The listing builds one solid part. Answer for the finished solid, in the listing's coordinates (mm). A direction names the side the tool comes from. Round coordinates to 2 decimals unless told otherwise and drop trailing zeros. Order: outer loops, then holes, each group sorted by start corner. A loop starts at its lowest first (then second) coordinate and runs counter-clockwise, first axis right, second up. Notation, with made-up numbers: M 36.25,64 L 63.25,64 A22 cw 63.25,100 Z; hole C 24,-9.75 d5. An arc over 180 degrees is marked long. Write item = value, one per line. Start each with the question number.
(1) A cutting plane is placed at C-C, the plane y = 39. Determine the outline of the cut face in (x, z), and give its area (3 significant figures).
(2) A cutting plane is placed at B-B, the plane y = 3. Determine the outline of the cut face in (x, z).
(3) Each of these flat-tipped pins is pushed along its axis until it touches: pin 1 (6 mm diameter, centred on x = 4.5, y = 12.5, fed in from +Z); pin 2 (4 mm diameter, centred on y = 6, z = -10, fed in from -X); pin 3 (6 mm diameter, centred on x = 20.5, z = -15.5, fed in from +Y); pin 4 (21 mm diameter, centred on x = 0, z = 0.02, fed in from +Y). Where does it stop, or does it pass through?
(4) Which of the six approach directions +Z, -Z, +X, -X, +Y, -Y give full straight-line access (tool end or side, diameter ignored) to faces 4 (the face through (0.75, 27.39, 15.5)), 5 (the face through (-7.27, 39.62, 23.09))?
(5) A cutting plane is placed at A-A, the plane z = 0. Determine the outline of the cut face in (x, y).
(6) Straight lines are drawn through the part: probe 1 along X at (y, z) = (13, 0.5); probe 2 along X at (y, z) = (22, 2.5); probe 3 along Z at (x, y) = (6, 44.5). For each, find the intervals that lie inside material, in ascending order. Write a range as from..to.
(7) For a pull along X with two mould halves and no side action, classify faces 1 (the face through (-2.08, 25.74, 23.65)), 2 (the face through (-30.736, 10.14, -4.036)), 3 (the face through (11, 46, 7)) as released by +X, released by -X, zero draft, split by the parting line, or undercut.
from build123d import *

# Parameters (mm, degrees)
M25X1_5_DI_LI_DELIK1_D     = 23.5
RADYUS1_R                  = 8
M10X1_0_DI_LI_DELIK2_D     = 9
M10X1_0_DI_LI_DELIK2_DEPTH = 10
M10X1_0_DI_LI_DELIK2_TIP   = 2.703872786


with BuildPart() as part:
    # Çizim1 → Döndür1 (revolve)
    with BuildSketch(Plane.XY, mode=Mode.PRIVATE) as d_nd_r1_sk:
        Polygon((0, 46), (0, 0), (31, 0), (31, 20), (22, 46), align=None)
    revolve(d_nd_r1_sk.sketch.rotate(Axis((0, 46, 0), (0, -1, 0)), 90), axis=Axis((0, 46, 0), (0, -1, 0)))

    # M25x1.5 Dişli Delik1 (through all)
    with Locations(Plane(origin=(0.000913764, 46, 0.015948363), x_dir=(0, 0, 1), z_dir=(0, 1, 0))):
        with Locations((0, 0)):
            Hole(M25X1_5_DI_LI_DELIK1_D / 2)

    # Radyus1
    radyus1_edges = [part.edges().sort_by_distance(p)[0] for p in [
        (0, 46, -22),
    ]]
    fillet(radyus1_edges, radius=RADYUS1_R)

    # M10x1.0 Dişli Delik2
    with Locations(Plane(origin=(0, 11.722589168, 33.865257596), x_dir=(1, 0, 0), z_dir=(0, 0.32711056388316634, 0.9449860734402582))):
        with Locations((0, 20.576424516)):
            Hole(M10X1_0_DI_LI_DELIK2_D / 2, depth=M10X1_0_DI_LI_DELIK2_DEPTH)
            with Locations((0, 0, -(M10X1_0_DI_LI_DELIK2_DEPTH + M10X1_0_DI_LI_DELIK2_TIP / 2))):  # 118° drill point
                Cone(0, M10X1_0_DI_LI_DELIK2_D / 2, M10X1_0_DI_LI_DELIK2_TIP, mode=Mode.SUBTRACT)

    # Çizim14 → Kes-Döndür1 (revolve, cut)
    with BuildSketch(Plane(origin=(0, 0, 0), x_dir=(0, 0, -1), z_dir=(1, 0, 0))):
        with BuildLine():
            Line((0, 0), (-18.203352341, 0))
            ThreePointArc((-18.203352341, 0), (-15.384211427, 1.092780017), (-12.5, 2))
            Line((-12.5, 2), (0, 2))
            Line((0, 2), (0, 0))
        make_face()
    revolve(axis=Axis((0, 0, 0), (0, 1, 0)), mode=Mode.SUBTRACT)


solid = part.part
Reported:
q1.outline = C 0,0 d48.85; hole C 0,0.02 d23.5
q1.area = 1,440 mm²
q2.outline = C 0,0 d62; hole C 0,0.02 d23.5
q3.pin_1 = 30.96
q3.pin_2 = -29.95
q3.pin_3 = 42.8
q3.pin_4 = through
q4.face_4 = none
q4.face_5 = +Y
q5.outline = M -31,0 L -18.2,0 A46.49 cw -12.5,2 L -11.75,2 L -11.75,46 L -16.3,46 A8 ccw -23.86,40.62 L -31,20 Z; M 11.75,2 L 12.5,2 A46.49 cw 18.2,0 L 31,0 L 31,20 L 23.86,40.62 A8 ccw 16.3,46 L 11.75,46 Z
q6.probe_1 = -31..-11.74, 11.74..31
q6.probe_2 = -30.2..-11.48, 11.49..30.2
q6.probe_3 = -20.09..-10.09, 10.12..20.09
q7.face_1 = undercut
q7.face_2 = split by the parting line
q7.face_3 = zero draft
